```python
from build123d import *

# Parameters (mm, degrees)
BOSS_EXTRUDE1_DEPTH = 10
SKETCH2_R           = 2
CUT_EXTRUDE1_DEPTH  = 52.590817981
SKETCH3_R           = 3.25
CUT_EXTRUDE2_DEPTH  = 6
FILLET1_R           = 5
SKETCH4_W           = 10
SKETCH4_H           = 20
BOSS_EXTRUDE2_DEPTH = 2
SKETCH5_W           = 10
SKETCH5_H           = 20
BOSS_EXTRUDE3_DEPTH = 2


with BuildPart() as part:
    # Sketch1 → Boss-Extrude1 (new body)
    with BuildSketch(Plane.XY):
        Polygon((0, 0), (0, -20.1), (20, -20.1), (20, 0), (46.45, 0), (46.45, 20), (-26.45, 20), (-26.45, 0), align=None)
    extrude(amount=BOSS_EXTRUDE1_DEPTH)

    # Sketch2 → Cut-Extrude1 (cut, through all)
    with BuildSketch(Plane.XY.offset(10)):
        with Locations((-22.2, 10)):
            Circle(SKETCH2_R)
        with Locations((10, -15.05)):
            Circle(SKETCH2_R)
        with Locations(Location((42.2, 10, 0), (0, 0, 180))):
            Circle(SKETCH2_R)
    extrude(amount=-CUT_EXTRUDE1_DEPTH, mode=Mode.SUBTRACT)

    # Sketch3 → Cut-Extrude2 (cut)
    with BuildSketch(Plane.XY.offset(10)):
        with Locations((-22.2, 10)):
            Circle(SKETCH3_R)
        with Locations((42.2, 10)):
            Circle(SKETCH3_R)
        with Locations((10, -15.05)):
            Circle(SKETCH3_R)
    extrude(amount=-CUT_EXTRUDE2_DEPTH, mode=Mode.SUBTRACT)

    # Fillet1
    fillet1_edges = [part.edges().sort_by_distance(p)[0] for p in [
        (20, 0, 5),
        (0, 0, 5),
    ]]
    fillet(fillet1_edges, radius=FILLET1_R)

    # Sketch4 → Boss-Extrude2 (add)
    with BuildSketch(Plane(origin=(46.45, 0, 0), x_dir=(0, 0, -1), z_dir=(1, 0, 0))):
        with Locations((-5, 10)):
            Rectangle(SKETCH4_W, SKETCH4_H)
    extrude(amount=BOSS_EXTRUDE2_DEPTH)

    # Sketch5 → Boss-Extrude3 (add)
    with BuildSketch(Plane.ZY.offset(26.45)):
        with Locations((5, 10)):
            Rectangle(SKETCH5_W, SKETCH5_H)
    extrude(amount=BOSS_EXTRUDE3_DEPTH)


solid = part.part
```
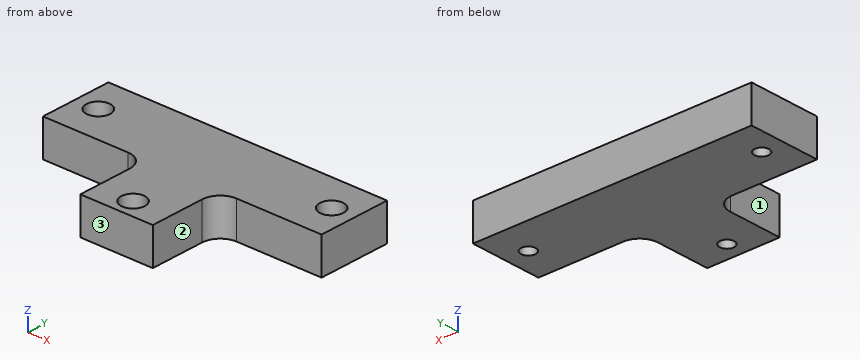
Source: CAD feature listing. Evaluate the final solid. Frame: model axes, mm. Face numbers are marked on the shaded views. A direction names the side the tool comes from. Give positions to 0.01 mm unless a question says otherwise; leave off trailing zeros. Loops run counter-clockwise (first coordinate to the right, second up) from the corner with the lowest first, then second, coordinate; pieces in that order, holes last. Notation, with made-up numbers: (68.25, 19.5) -> (127.25, 19.5) arc R24 ccw to (127.25, 35.5) -> close; hole circle Ø9 at (-13.5, 84). An arc over 180 degrees is marked (long way). Put each result on its own line as item: value. Start each with the question number.
1) Cut plane A-A (x = 42.2). Return loops of the section in (y, z), then the cut area to 3 significant figures.
2) Cut plane C-C (z = 4.75). Return loops of the section in (x, y).
3) Cut plane D-D (y = 10). Return loops of the section in (x, z), then the cut area to 3 significant figures.
4) Reachability of the marked faces 1, 2 and 3 from +Z, -Z, +X, -X, +Y, -Y: full face, straight path, thin tool, end or side. Return the list, or none.
5) Contact query for flat-ended pins moving along their axis: P1, Ø3, axis at y = -12.5, z = 6, coming from the -X side; P2, Ø1.5, axis at x = 25.5, z = 8.5, coming from the -Y side; P3, Ø5, axis at y = -15, z = 5, coming from the +X side; P4, Ø3.5, axis at x = -22.2, y = 10, coming from the +Z side. Output: stop coordinate, or through.
6) Material intervals for probe 1 along Y at (x, z) = (10, 6.1); probe 2 along Y at (x, z) = (42.2, 2.7); probe 3 along Y at (x, z) = (-16, 6.25), sorted ascending.
Results are:
1. outline: (0, 0) -> (8, 0) -> (8, 4) -> (6.75, 4) -> (6.75, 10) -> (0, 10) -> close; (12, 0) -> (20, 0) -> (20, 10) -> (13.25, 10) -> (13.25, 4) -> (12, 4) -> close
1. area: 145 mm2
2. outline: (-28.45, 0) -> (-5, 0) arc R5 cw to (0, -5) -> (0, -20.1) -> (20, -20.1) -> (20, -5) arc R5 cw to (25, 0) -> (48.45, 0) -> (48.45, 20) -> (-28.45, 20) -> close; hole circle Ø6.5 at (-22.2, 10); hole circle Ø6.5 at (10, -15.05); hole circle Ø6.5 at (42.2, 10)
3. outline: (-28.45, 0) -> (-24.2, 0) -> (-24.2, 4) -> (-25.45, 4) -> (-25.45, 10) -> (-28.45, 10) -> close; (-20.2, 0) -> (40.2, 0) -> (40.2, 4) -> (38.95, 4) -> (38.95, 10) -> (-18.95, 10) -> (-18.95, 4) -> (-20.2, 4) -> close; (44.2, 0) -> (48.45, 0) -> (48.45, 10) -> (45.45, 10) -> (45.45, 4) -> (44.2, 4) -> close
3. area: 659 mm2
4. face 1: +Z, -Z, -X, -Y
4. face 2: +Z, -Z, +X, -Y
4. face 3: +Z, -Z, +X, -X, -Y
5. P1: stops at x = 0
5. P2: stops at y = -0.01
5. P3: stops at x = 20
5. P4: passes through
6. probe 1: y = -20.1 to -18.3, -11.8 to 20
6. probe 2: y = 0 to 8, 12 to 20
6. probe 3: y = 0 to 20
